Design review of the part shown in the three views and the two pictorial views. Dimensions are in mm from the part's minimum x, y and z. A direction names the side the tool comes from. Give positions to 0.01 mm unless a question says otherwise; leave off trailing zeros. Write each loop counter-clockwise with the first axis right and the second up, starting at its lowest first coordinate (ties: lowest second). Pieces come first, ordered by that corner, then holes. Notation, with made-up numbers: (24, 28) -> (62, 28) arc R19 ccw to (62, 36) -> close; hole circle Ø11 at (-2, 65). An arc over 180 degrees is marked (long way). Return JSON: item names as keys, results as strings. Group by question number.
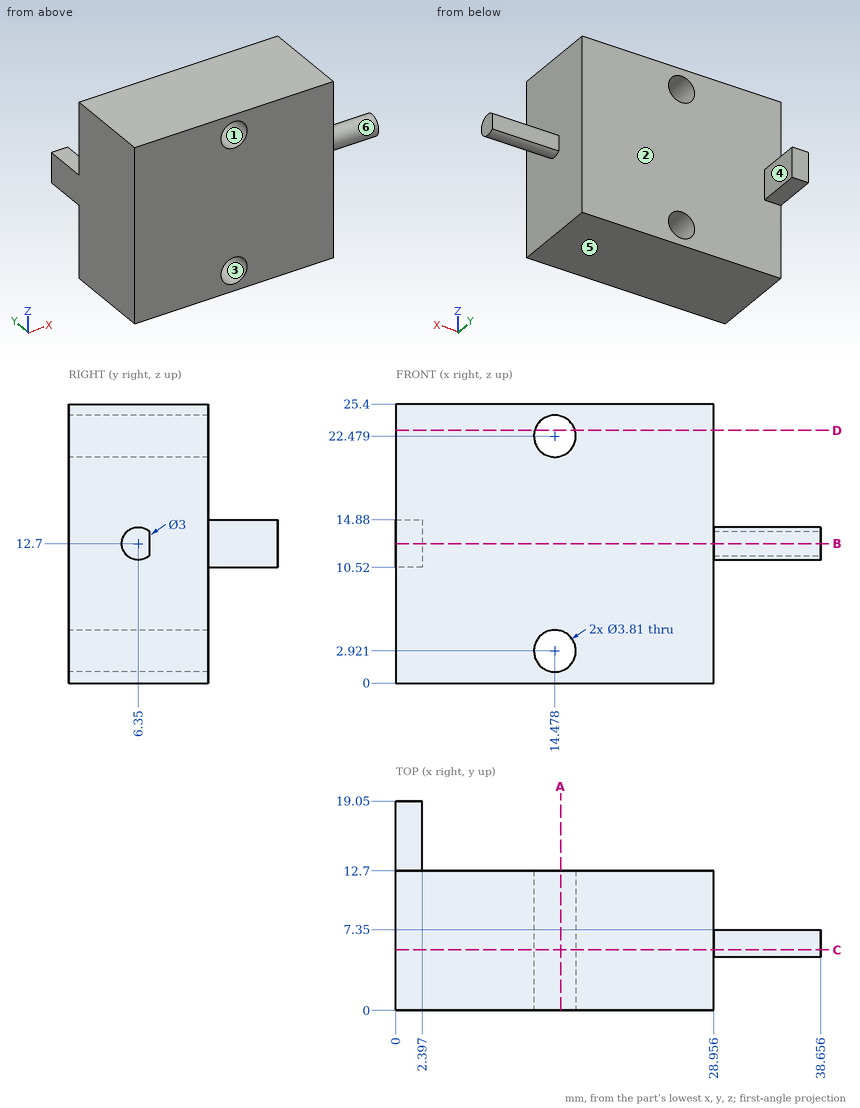
Q1. For L1, parallel to X at y = 8.75, z = 3 (1 decimal); L2, parallel to Z at x = 14, y = 1.5 (1 decimal); L3, parallel to X at y = 17.25, z = 14, list the stretches that pass through material, from the lowest coordinate up. Write a range as from..to.
Q2. Take a section at B-B, the plane z = 12.7. Give the boundary of the cut face in (x, y), plus the area to 3 significant figures.
Q3. Insertion check: pin 1 (3 mm diameter, centred on x = 14.478, z = 2.921, fed in from -Y); pin 2 (12.5 mm diameter, centred on x = 20.5, z = 13, fed in from +Y); pin 3 (1.9 mm diameter, centred on x = 0.5, y = 14.5, fed in from -Z); pin 4 (0.7 mm diameter, centred on x = 34, z = 12.5, fed in from +Y). Each pin has a flat end and moves straight along its axis. Give the tip position at first contact, or say it passes through.
Q4. Tool access review of the marked faces 5 and 6: name each direction out of +Z, -Z, +X, -X, +Y, -Y from which nothing blocks a thin tool from reaching the whole face with its end or side.
Q5. Take a section at C-C, the plane y = 5.5. Give the boundary of the cut face in (x, z) (1 decimal).
Q6. Mouldability with a two-part tool opening along X and no side actions: class the marked faces 1, 2, 3 and 4 as +X half, -X half, draft (parallel to the pull), parting line (faces both ways), or undercut.
Q7. Take a section at D-D, the plane z = 23. Give the boundary of the cut face in (x, y) (1 decimal).
Q8. Take a section at A-A, the plane x = 15. Give the boundary of the cut face in (y, z).
Final values:
{
 "1": {"L1": "x = 0..12.6, 16.4..29", "L2": "z = 0..1.1, 4.8..20.6, 24.3..25.4", "L3": "x = 0..2.4"},
 "2": {"outline": "(0, 0) -> (28.96, 0) -> (28.96, 4.85) -> (38.66, 4.85) -> (38.66, 7.35) -> (28.96, 7.35) -> (28.96, 12.7) -> (2.4, 12.7) -> (2.4, 19.05) -> (0, 19.05) -> close", "area": "407 mm²"},
 "3": {"pin 1": "passes through", "pin 2": "stops at y = 12.7", "pin 3": "stops at z = 10.52", "pin 4": "stops at y = 7.35"},
 "4": {"face 5": "-Z, +X, -X, +Y, -Y", "face 6": "+X"},
 "5": {"outline": "(0, 0) -> (29, 0) -> (29, 11.5) -> (38.7, 11.5) -> (38.7, 13.9) -> (29, 13.9) -> (29, 25.4) -> (0, 25.4) -> close; hole circle Ø3.8 at (14.5, 2.9); hole circle Ø3.8 at (14.5, 22.5)"},
 "6": {"face 1": "undercut", "face 2": "draft", "face 3": "undercut", "face 4": "+X half"},
 "7": {"outline": "(0, 0) -> (12.6, 0) -> (12.6, 12.7) -> (0, 12.7) -> close; (16.3, 0) -> (29, 0) -> (29, 12.7) -> (16.3, 12.7) -> close"},
 "8": {"outline": "(0, 0) -> (12.7, 0) -> (12.7, 1.09) -> (0, 1.09) -> close; (0, 4.75) -> (12.7, 4.75) -> (12.7, 20.65) -> (0, 20.65) -> close; (0, 24.31) -> (12.7, 24.31) -> (12.7, 25.4) -> (0, 25.4) -> close"}
}
